Check sheet for the modelled part. Datum: model origin and axes. Units: mm. Face numbers are marked on the shaded views. A direction names the side the tool comes from. Round coordinates to 2 decimals unless told otherwise and drop trailing zeros. Loops run counter-clockwise (first coordinate to the right, second up) from the corner with the lowest first, then second, coordinate; pieces in that order, holes last. Notation, with made-up numbers: M 25.5,19.25 L 42.5,19.25 A20 ccw 42.5,43.25 Z; hole C 22,74.5 d10. An arc over 180 degrees is marked long. One line per question, with ' | ' between items. Start each with the question number.
(1) Go/stop test with flat-tipped pins: P1, Ø5.5, axis at y = 6.5, z = 10.5, coming from the -X side; P2, Ø2, axis at y = 11, z = -6, coming from the +X side; P3, Ø8.5, axis at x = 11.5, z = -4, coming from the +Y side; P4, Ø11, axis at x = 14, z = 0, coming from the +Y side. Record where each tip stops, or that it passes through.
(2) Section check D-D (y = -8.5). Record the boundary of the cut face in (x, z), and give its area (3 significant figures).
(3) Section check A-A (y = 0). Record the boundary of the cut face in (x, z).
(4) Tool access check on the marked faces 1, 2 and 3. Record the directions out of +Z, -Z, +X, -X, +Y, -Y that give a thin tool (end or side, any length) a straight path to the whole face; none if there is none.
(5) Section check C-C (x = -23). Record the boundary of the cut face in (y, z).
(6) Thickness scan on probe 1 along Y at (x, z) = (-22, 2); probe 2 along X at (y, z) = (5.25, -1.5). Record the ranges inside material, lowest first. Write a range as [from, to].
(7) Section check B-B (z = 0). Record the boundary of the cut face in (x, y), and give its area (3 significant figures).
(8) Draft check along X on the marked faces 4, 5 and 6. Enter one of: +X half, -X half, draft (parallel to the pull), parting line (faces both ways), or undercut.
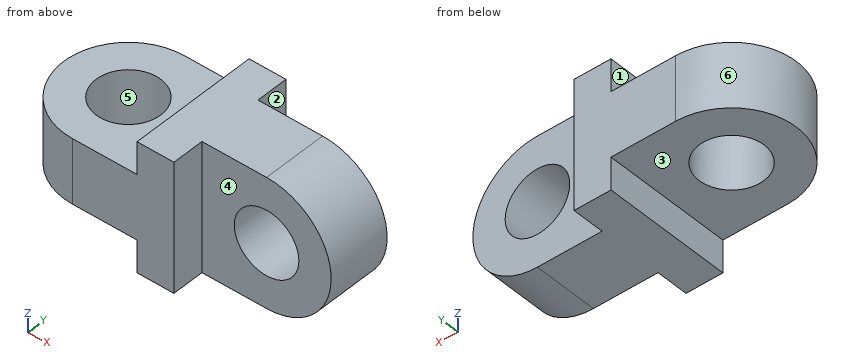
```python
from build123d import *

# Parameters (mm, degrees)
SKETCH1_R           = 7
BOSS_EXTRUDE1_DEPTH = 7
SKETCH2_W           = 28
SKETCH2_H           = 28
BOSS_EXTRUDE2_DEPTH = 8
SKETCH3_R           = 7
BOSS_EXTRUDE3_DEPTH = 7


with BuildPart() as part:
    # Sketch1 → Boss-Extrude1 (new body, symmetric)
    with BuildSketch(Plane(origin=(0, 0, 0), x_dir=(1, 0, 0), z_dir=(0, 1, 0))):
        with BuildLine():
            Line((0, 14), (0, -14))
            Line((0, -14), (14, -14))
            ThreePointArc((14, -14), (28, 0), (14, 14))
            Line((14, 14), (0, 14))
        make_face()
        with Locations((14, 0)):
            Circle(SKETCH1_R, mode=Mode.SUBTRACT)
    extrude(amount=BOSS_EXTRUDE1_DEPTH, both=True)

    # Sketch2 → Boss-Extrude2 (add)
    with BuildSketch(Plane.ZY):
        Rectangle(SKETCH2_W, SKETCH2_H)
    extrude(amount=BOSS_EXTRUDE2_DEPTH)

    # Sketch3 → Boss-Extrude3 (add, symmetric)
    with BuildSketch(Plane(origin=(0, 0, 0), x_dir=(-1, 0, 0), z_dir=(0, 0, -1))):
        with BuildLine():
            Line((8, 14), (8, -14))
            Line((8, -14), (22, -14))
            ThreePointArc((22, -14), (36, 0), (22, 14))
            Line((22, 14), (8, 14))
        make_face()
        with Locations((22, 0)):
            Circle(SKETCH3_R, mode=Mode.SUBTRACT)
    extrude(amount=BOSS_EXTRUDE3_DEPTH, both=True)


solid = part.part
```
The answers:
1) P1: x = -8 | P2: x = 0 | P3: y = 7 | P4: through
2) outline: M -33.12,-7 L -8,-7 L -8,-14 L 0,-14 L 0,14 L -8,14 L -8,7 L -33.12,7 Z | area: 576 mm²
3) outline: M -36,-7 L -29,-7 L -29,7 L -36,7 Z; M -15,-7 L -8,-7 L -8,-14 L 14,-14 A14 ccw 14,14 L -8,14 L -8,7 L -15,7 Z; hole C 14,0 d14
4) face 1: +Z, -X, +Y, -Y | face 2: +Z, -Z, +X, +Y | face 3: -Z, -X, +Y, -Y
5) outline: M -13.96,-7 L -6.93,-7 L -6.93,7 L -13.96,7 Z; M 6.93,-7 L 13.96,-7 L 13.96,7 L 6.93,7 Z
6) probe 1: [-14, -7], [7, 14] | probe 2: [-34.98, -26.63], [-17.37, 7.16], [20.84, 27.92]
7) outline: M -22,-14 L 0,-14 L 0,-7 L 7,-7 L 7,7 L 0,7 L 0,14 L -22,14 A14 ccw Z; M 21,-7 L 28,-7 L 28,7 L 21,7 Z; hole C -22,0 d14 | area: 966 mm²
8) face 4: draft | face 5: undercut | face 6: -X half
